Check sheet for the modelled part. Datum: model origin and axes. Units: mm. A direction names the side the tool comes from. Coordinates: 2 decimals unless noted, no trailing zeros. Order: outer loops, then holes, each group sorted by start corner. A loop starts at its lowest first (then second) coordinate and runs counter-clockwise, first axis right, second up.
1. Cross-section at D-D (y = -1.5). Enter the section's corners in (x, z).
2. Cross-section at C-C (x = -41). Enter the section's corners in (y, z).
3. Set-up check for faces 1 (the flat face through (56, -5, 0)), 2 (the flat face through (-56, -5, 0)), 3 (the cylindrical face through (56.268, 86.583, 7.759)): record each of +Z, -Z, +X, -X, +Y, -Y from which the full face is reachable in a straight line by a thin tool's end or side.
4. Draft check along X on faces 4 (the flat face through (-1, 53, 22.5)), 5 (the flat face through (1, 112, -23.2)), 6 (the flat face through (-57.5, 59, 0)), 7 (the flat face through (-1, 32, -25)). Enter one of: released by +X, released by -X, zero draft, split by the parting line, or undercut.
5. Gauge pin test, flat ends, axial feed: pin 1 Ø6 at (x, z) = (36.5, -15) entering from -Y; pin 2 Ø18.5 at (x, y) = (-7.5, 97.5) entering from -Z; pin 3 Ø11 at (y, z) = (90, 7) entering from +X; pin 4 Ø1.4 at (x, z) = (2, -24.5) entering from -Y. Record the tip position at first contact, or that the pin passes through.
6. Cross-section at A-A (y = 90). Enter the section's corners in (x, z), then the cut area to 3 significant figures.
7. Thickness scan on line 1 (Z direction, x = 49.5, y = 36.5); line 2 (X direction, y = 45.5, z = 15); line 3 (X direction, y = -1.5, z = 9.5). Record the ranges inside material, lowest first.
8. Cross-section at B-B (z = 7). Enter the section's corners in (x, y), then the cut area to 4 significant figures.
```python
from build123d import *

# Parameters (mm, degrees)
SKETCH_1_W          = 115
SKETCH_1_H          = 50
EXTRUDE_1_DEPTH     = 120
SKETCH_4_W          = 86
SKETCH_4_H          = 44
CUT_EXTRUDE_3_DEPTH = 28
SKETCH_6_W          = 102
SKETCH_6_H          = 61
CUT_EXTRUDE_4_DEPTH = 1.8
SKETCH_8_W          = 112
SKETCH_8_H          = 47
EXTRUDE_3_DEPTH     = 10
SKETCH_10_W         = 110
SKETCH_10_H         = 44
CUT_EXTRUDE_5_DEPTH = 127
SKETCH_11_R         = 3.5
CUT_EXTRUDE_6_DEPTH = 10


with BuildPart() as part:
    # 草图1 → 凸台-拉伸1 (new body)
    with BuildSketch(Plane(origin=(0, 0, 0), x_dir=(1, 0, 0), z_dir=(0, 1, 0))):
        Rectangle(SKETCH_1_W, SKETCH_1_H)
    extrude(amount=EXTRUDE_1_DEPTH)

    # 草图4 → 切除-拉伸3 (cut)
    with BuildSketch(Plane(origin=(0, 0, -25), x_dir=(-1, 0, 0), z_dir=(0, 0, -1))):
        with Locations((0, 84.556060941)):
            Rectangle(SKETCH_4_W, SKETCH_4_H)
    extrude(amount=-CUT_EXTRUDE_3_DEPTH, mode=Mode.SUBTRACT)

    # 草图6 → 切除-拉伸4 (cut)
    with BuildSketch(Plane(origin=(0, 0, -25), x_dir=(-1, 0, 0), z_dir=(0, 0, -1))):
        with Locations((0, 84.556060941)):
            Rectangle(SKETCH_6_W, SKETCH_6_H)
    extrude(amount=-CUT_EXTRUDE_4_DEPTH, mode=Mode.SUBTRACT)

    # 草图8 → 凸台-拉伸3 (add)
    with BuildSketch(Plane.XZ):
        Rectangle(SKETCH_8_W, SKETCH_8_H)
    extrude(amount=EXTRUDE_3_DEPTH)

    # 草图10 → 切除-拉伸5 (cut)
    with BuildSketch(Plane.XZ.offset(10)):
        with Locations((0, 0.5)):
            Rectangle(SKETCH_10_W, SKETCH_10_H)
    extrude(amount=-CUT_EXTRUDE_5_DEPTH, mode=Mode.SUBTRACT)

    # 草图11 → 切除-拉伸6 (cut)
    with BuildSketch(Plane(origin=(57.5, 0, 0), x_dir=(0, 0, -1), z_dir=(1, 0, 0))):
        with Locations((-7, 90)):
            Circle(SKETCH_11_R)
    extrude(amount=-CUT_EXTRUDE_6_DEPTH, mode=Mode.SUBTRACT)


solid = part.part
```
Data:
1. outline: (-56, -23.5) - (56, -23.5) - (56, 23.5) - (-56, 23.5) - close; hole (-55, -21.5) - (55, -21.5) - (55, 22.5) - (-55, 22.5) - close
2. outline: (-10, -23.5) - (0, -23.5) - (0, -25) - (54.06, -25) - (54.06, -23.2) - (62.56, -23.2) - (62.56, -21.5) - (-10, -21.5) - close; (-10, 22.5) - (117, 22.5) - (117, -21.5) - (106.56, -21.5) - (106.56, -23.2) - (115.06, -23.2) - (115.06, -25) - (120, -25) - (120, 25) - (0, 25) - (0, 23.5) - (-10, 23.5) - close
3. face 1: +Z, -Z, +X, -Y
3. face 2: +Z, -Z, -X, -Y
3. face 3: +X
4. face 4: undercut
4. face 5: undercut
4. face 6: released by -X
4. face 7: zero draft
5. pin 1: stops at y = 117
5. pin 2: stops at z = -23.2
5. pin 3: stops at x = 57.5
5. pin 4: stops at y = 0
6. outline: (-57.5, -25) - (-51, -25) - (-51, -23.2) - (-43, -23.2) - (-43, -21.5) - (-55, -21.5) - (-55, 22.5) - (55, 22.5) - (55, 10.5) - (57.5, 10.5) - (57.5, 25) - (-57.5, 25) - close; (43, -23.2) - (51, -23.2) - (51, -25) - (57.5, -25) - (57.5, 3.5) - (55, 3.5) - (55, -21.5) - (43, -21.5) - close
6. area: 563 mm2
7. line 1: z = -25 to -21.5, 22.5 to 25
7. line 2: x = -57.5 to -55, 55 to 57.5
7. line 3: x = -56 to -55, 55 to 56
8. outline: (-57.5, 0) - (-56, 0) - (-56, -10) - (-55, -10) - (-55, 117) - (55, 117) - (55, 93.5) - (57.5, 93.5) - (57.5, 120) - (-57.5, 120) - close; (55, -10) - (56, -10) - (56, 0) - (57.5, 0) - (57.5, 86.5) - (55, 86.5) - close
8. area: 932.5 mm2
